```python
from build123d import *

# Parameters (mm, degrees)
SCHIZZO3_R               = 3
TAGLIO_ESTRUSIONE1_DEPTH = 15
RACCORDO1_R              = 1


with BuildPart() as part:
    # Schizzo2 → Rivoluzione1 (revolve)
    with BuildSketch(Plane.XY, mode=Mode.PRIVATE) as rivoluzione1_sk:
        Polygon((0, 0), (11, 0), (10, 17), (0, 17), align=None)
    revolve(rivoluzione1_sk.sketch.rotate(Axis((0, 17, 0), (0, -1, 0)), 180), axis=Axis((0, 17, 0), (0, -1, 0)))

    # Schizzo3 → Taglio-Estrusione1 (cut)
    with BuildSketch(Plane.XZ):
        Circle(SCHIZZO3_R)
    extrude(amount=-TAGLIO_ESTRUSIONE1_DEPTH, mode=Mode.SUBTRACT)

    # Raccordo1
    raccordo1_edges = [part.edges().sort_by_distance(p)[0] for p in [
        (10, 17, 0),
    ]]
    fillet(raccordo1_edges, radius=RACCORDO1_R)


solid = part.part
```
Geometry check sheet. Reference: the model listing, model coordinates, mm. A direction names the side the tool comes from. Give positions to 0.01 mm unless a question says otherwise; leave off trailing zeros. Order: outer loops, then holes, each group sorted by start corner. A loop starts at its lowest first (then second) coordinate and runs counter-clockwise, first axis right, second up. Notation, with made-up numbers: (67, 76.25) - (102, 76.25) arc R11 ccw to (102, 97.25) - close; hole circle Ø9 at (2.5, 14). An arc over 180 degrees is marked (long way). Answer in a Markdown table with one row per item. Add a question column.
Q1. Mould release check, pull along X, two halves, no side actions. Record for faces 3 (the flat face through (2.3, 0, 2.3)), 4 (the cylindrical face through (-3, 7, 0)), 5 (the conical face through (8.35, 8.14, 6.4)): pulls with the +X half, pulls with the -X half, needs draft (parallel to the pull), parting line crosses it, or undercut.
Q2. Material ranges on probe 1 along Z at (x, y) = (0, 3.25); probe 2 along Z at (x, y) = (0, 7.5); probe 3 along Y at (x, z) = (0, 1.25), recorded low to high. Write a range as from..to.
Q3. Cross-section at B-B, the plane x = 0. Enter the section's corners in (y, z).
Q4. Gauge pin test, flat ends, axial feed: pin 1 (6 mm diameter, centred on x = 2, z = -7, fed in from -Y); pin 2 (5 mm diameter, centred on x = 1, y = 3.5, fed in from +Z); pin 3 (6 mm diameter, centred on x = 4.5, y = 12.5, fed in from +Z); pin 4 (4 mm diameter, centred on y = 15, z = 5.5, fed in from +X). Record the tip position at first contact, or that the pin passes through.
Q5. Cross-section at A-A, the plane z = 0. Enter the section's corners in (x, y).
Q6. Cross-section at D-D, the plane y = 5.5. Enter the section's corners in (x, z), then the cut area to 3 significant figures.
Q7. Tool access check on faces 1 (the flat face through (0, 15, 0)), 2 (the flat face through (0, 17, 0)). Record the directions out of +Z, -Z, +X, -X, +Y, -Y that give a thin tool (end or side, any length) a straight path to the whole face; none if there is none.
Q8. Cross-section at C-C, the plane y = 8.75. Enter the section's corners in (x, z), then the cut area to 3 significant figures.
Check values:
| question | item | result |
|---|---|---|
| 1 | face 3 | needs draft |
| 1 | face 4 | undercut |
| 1 | face 5 | parting line crosses it |
| 2 | probe 1 | z = -10.81..-3, 3..10.81 |
| 2 | probe 2 | z = -10.56..-3, 3..10.56 |
| 2 | probe 3 | y = 15..17 |
| 3 | outline | (0, -11) - (16.06, -10.06) arc R1 ccw to (17, -9.06) - (17, 9.06) arc R1 ccw to (16.06, 10.06) - (0, 11) - (0, 3) - (15, 3) - (15, -3) - (0, -3) - close |
| 4 | pin 1 | stops at y = 0 |
| 4 | pin 2 | stops at z = 10.93 |
| 4 | pin 3 | stops at z = 10.19 |
| 4 | pin 4 | stops at x = 9.5 |
| 5 | outline | (-11, 0) - (-3, 0) - (-3, 15) - (3, 15) - (3, 0) - (11, 0) - (10.06, 16.06) arc R1 ccw to (9.06, 17) - (-9.06, 17) arc R1 ccw to (-10.06, 16.06) - close |
| 6 | outline | circle Ø21.35 at (0, 0); hole circle Ø6 at (0, 0) |
| 6 | area | 330 mm^2 |
| 7 | face 1 | -Y |
| 7 | face 2 | +Z, -Z, +X, -X, +Y |
| 8 | outline | circle Ø20.97 at (0, 0); hole circle Ø6 at (0, 0) |
| 8 | area | 317 mm^2 |
